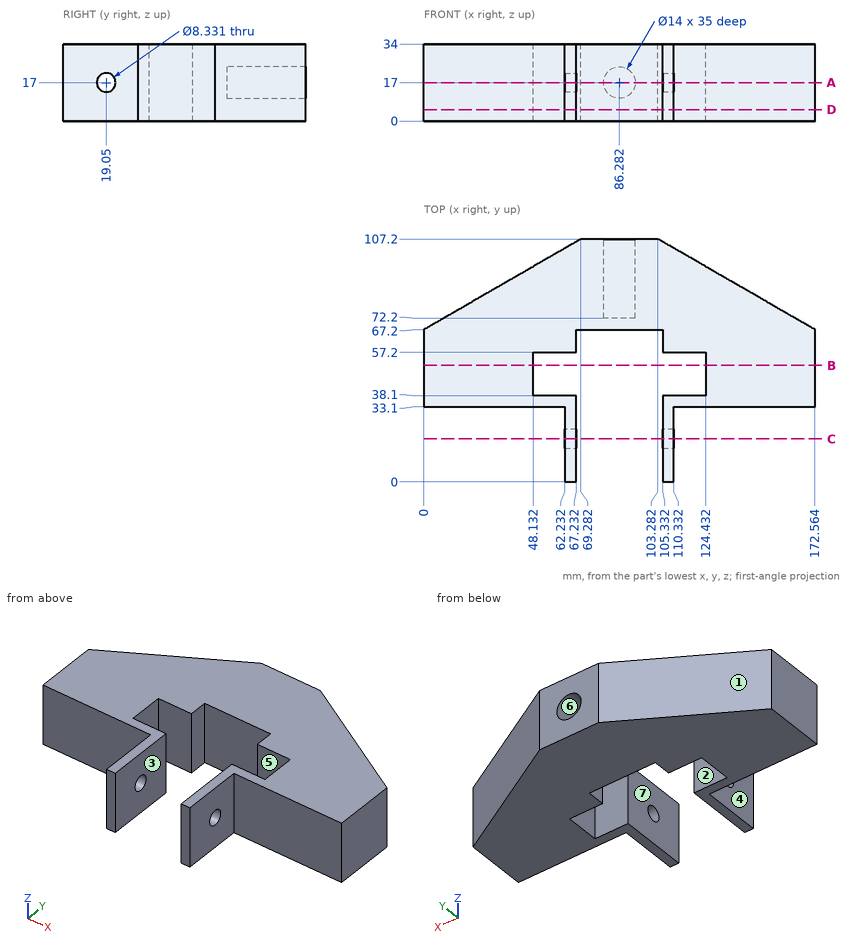
Source: three-view drawing plus pictorial views. Frame: mm from the lowest corner of the part. A direction names the side the tool comes from. Coordinates: 2 decimals unless noted, no trailing zeros. Order: outer loops, then holes, each group sorted by start corner. A loop starts at its lowest first (then second) coordinate and runs counter-clockwise, first axis right, second up.
Item 1: Pull-direction query (Y, two-part tool) for the marked faces 1, 2 and 3; classes: pulls with the +Y half, pulls with the -Y half, needs draft (parallel to the pull), parting line crosses it, or undercut.
Output values:
face 1: pulls with the +Y half
face 2: undercut
face 3: needs draft
Item 2: Cut plane D-D (z = 5). Return loops of the section in (x, y), plus the area to 3 significant figures.
Output values:
outline: (0, 33.1) - (62.23, 33.1) - (62.23, 0) - (67.23, 0) - (67.23, 38.1) - (48.13, 38.1) - (48.13, 57.2) - (67.23, 57.2) - (67.23, 67.2) - (105.33, 67.2) - (105.33, 57.2) - (124.43, 57.2) - (124.43, 38.1) - (105.33, 38.1) - (105.33, 0) - (110.33, 0) - (110.33, 33.1) - (172.56, 33.1) - (172.56, 67.2) - (103.28, 107.2) - (69.28, 107.2) - (0, 67.2) - close
area: 8,320 mm2
Item 3: Set-up query: the marked faces 4, 5, 6 and 7. Return all of +Z, -Z, +X, -X, +Y, -Y with unobstructed straight access to the full face (end or side cutting, diameter ignored); none if empty.
Output values:
face 4: +Z, -Z, -X, -Y
face 5: +Z, -Z
face 6: +Y
face 7: +Z, -Z, -Y
Item 4: First-contact query: P1, Ø10, axis at y = 15, z = 21, coming from the -X side; P2, Ø1.5, axis at y = 88, z = 22, coming from the -X side; P3, Ø5.5, axis at x = 61.5, z = 20.5, coming from the +Y side (1 decimal). Flat tips, straight axial feed; report the tip coordinate or a pass-through.
Output values:
P1: stops at x = 62.23
P2: stops at x = 34.73
P3: stops at y = 104.3
Item 5: Cut plane B-B (y = 51.5). Return loops of the section in (x, z).
Output values:
outline: (0, 0) - (48.13, 0) - (48.13, 34) - (0, 34) - close; (124.43, 0) - (172.56, 0) - (172.56, 34) - (124.43, 34) - close
Item 6: Cut plane C-C (y = 19.05). Return loops of the section in (x, z).
Output values:
outline: (62.23, 0) - (67.23, 0) - (67.23, 12.83) - (62.23, 12.83) - close; (62.23, 21.17) - (67.23, 21.17) - (67.23, 34) - (62.23, 34) - close; (105.33, 0) - (110.33, 0) - (110.33, 12.83) - (105.33, 12.83) - close; (105.33, 21.17) - (110.33, 21.17) - (110.33, 34) - (105.33, 34) - close
Item 7: Material intervals for line 1 (X direction, y = 34.5, z = 8); line 2 (X direction, y = 38.5, z = 19.5); line 3 (Z direction, x = 106.5, y = 19.05), sorted ascending.
Output values:
line 1: x = 0 to 67.23, 105.33 to 172.56
line 2: x = 0 to 48.13, 124.43 to 172.56
line 3: z = 0 to 12.83, 21.17 to 34
Item 8: Cut plane A-A (z = 17). Count the separate pieces of the cut face and the enclosed holes in it, plus the area to 3 significant figures.
Output values:
separate pieces: 3
enclosed holes: 0
area: 7,740 mm2
